```python
from build123d import *

# Parameters (mm, degrees)
BOSS_EXTRUDE1_DEPTH     = 40
CUT_EXTRUDE1_DEPTH      = 20
CUT_EXTRUDE1_DEPTH_BACK = 20
SKETCH2_R               = 1.7
BOSS_EXTRUDE2_START     = -3
SKETCH4_W               = 64
SKETCH4_H               = 30
SKETCH4_R               = 2
BOSS_EXTRUDE2_DEPTH     = 3
FILLET1_R               = 1
BOSS_EXTRUDE3_START     = -3
BOSS_EXTRUDE3_DEPTH     = 3
FILLET2_R               = 2
BOSS_EXTRUDE4_START     = -2
BOSS_EXTRUDE4_DEPTH     = 2
CHAMFER1_SIZE           = 4
CHAMFER3_SIZE           = 4
FILLET3_R               = 2


with BuildPart() as part:
    # Sketch1 → Boss-Extrude1 (new body)
    with BuildSketch(Plane.XY):
        Polygon((-3, -3), (-3, 15), (0, 15), (0, 0), (15.4, 0), (15.4, 15), (18.4, 15), (18.4, -3), align=None)
    extrude(amount=BOSS_EXTRUDE1_DEPTH)

    # Sketch2 → Cut-Extrude1 (cut, two sides: drawn at the far end of the back side and taken through both)
    with BuildSketch(Plane(origin=(0, 0, 0), x_dir=(0, 0, -1), z_dir=(1, 0, 0)).offset(-CUT_EXTRUDE1_DEPTH_BACK)):
        with Locations(Location((-34, 7.5, 0), (0, 0, 180))):
            Circle(SKETCH2_R)
        with Locations(Location((-9, 7.5, 0), (0, 0, 180))):
            Circle(SKETCH2_R)
    extrude(amount=CUT_EXTRUDE1_DEPTH + CUT_EXTRUDE1_DEPTH_BACK, mode=Mode.SUBTRACT)

    # Sketch4 → Boss-Extrude2 (add)
    with BuildSketch(Plane(origin=(0, 0, 0), x_dir=(-1, 0, 0), z_dir=(0, 0, -1)).offset(BOSS_EXTRUDE2_START)):
        with Locations((-29, -18)):
            Rectangle(SKETCH4_W, SKETCH4_H)
        with Locations((-4.875030798, -23.000128049)):
            Circle(SKETCH4_R, mode=Mode.SUBTRACT)
        with Locations((-4.87501026, -12.999951056)):
            Circle(SKETCH4_R, mode=Mode.SUBTRACT)
        with Locations((-53.124974567, -23.00004902)):
            Circle(SKETCH4_R, mode=Mode.SUBTRACT)
        with Locations((-53.125010259, -12.999787804)):
            Circle(SKETCH4_R, mode=Mode.SUBTRACT)
        with BuildLine():
            Line((-1.999964331, -28.999999992), (-55.999999981, -28.997992053))
            Line((-55.999999981, -28.997992053), (-51.282852208, -26.550624356))
            ThreePointArc((-51.282852208, -26.550624356), (-49.706744703, -25.077476419), (-49.124974567, -23.00004902))
            Line((-49.124974567, -23.00004902), (-49.125010259, -12.999787804))
            ThreePointArc((-49.125010259, -12.999787804), (-49.706039872, -10.923579364), (-51.280331003, -9.450540216))
            Line((-51.280331003, -9.450540216), (-55.999146244, -6.99799207))
            Line((-55.999146244, -6.99799207), (-1.999146282, -7.000000007))
            Line((-1.999146282, -7.000000007), (-6.718065019, -9.449859627))
            ThreePointArc((-6.718065019, -9.449859627), (-8.293505472, -10.922960328), (-8.87501026, -12.999951056))
            Line((-8.87501026, -12.999951056), (-8.875030798, -23.000128049))
            ThreePointArc((-8.875030798, -23.000128049), (-8.293584076, -25.077023205), (-6.718284054, -26.550116421))
            Line((-6.718284054, -26.550116421), (-1.999964331, -28.999999992))
        make_face(mode=Mode.SUBTRACT)
    extrude(amount=BOSS_EXTRUDE2_DEPTH)

    # Fillet1
    fillet1_edges = [part.edges().sort_by_distance(p)[0] for p in [
        (55.999999981, -28.997992053, 1.5),
        (1.999964331, -28.999999992, 1.5),
        (1.999146282, -7.000000007, 1.5),
        (55.999146244, -6.99799207, 1.5),
    ]]
    fillet(fillet1_edges, radius=FILLET1_R)

    # Sketch6 → Boss-Extrude3 (add)
    with BuildSketch(Plane(origin=(0, 0, 0), x_dir=(-1, 0, 0), z_dir=(0, 0, -1)).offset(BOSS_EXTRUDE3_START)):
        Polygon((-18.4, 15), (-61, -3), (-18.4, -3), align=None)
    extrude(amount=BOSS_EXTRUDE3_DEPTH)

    # Fillet2
    fillet2_edges = [part.edges().sort_by_distance(p)[0] for p in [
        (61, -3, 1.5),
        (-3, -33, 1.5),
        (61, -33, 1.5),
    ]]
    fillet(fillet2_edges, radius=FILLET2_R)

    # Sketch7 → Boss-Extrude4 (add)
    with BuildSketch(Plane.ZY.offset(3).offset(BOSS_EXTRUDE4_START)):
        Polygon((3, -17), (14.5, -3), (3, -3), align=None)
    extrude(amount=BOSS_EXTRUDE4_DEPTH)

    # Chamfer1
    # the kernel refuses this chamfer: 4 mm, written as the material it takes off along each edge
    with BuildSketch(Plane(origin=(28.686731952, -3, 40), x_dir=(0, -0.027495876610586403, -0.9996219169112968), z_dir=(-1, 0, 0))) as chamfer1_piece_1:
        Polygon((CHAMFER1_SIZE * 0.999621916911, -CHAMFER1_SIZE * 0.0274958766106), (-CHAMFER1_SIZE * 0.0274958766106, -CHAMFER1_SIZE * 0.999621916911), (0, 0), align=None)
    extrude(amount=41.973463904, mode=Mode.SUBTRACT)

    # Chamfer3
    chamfer3_edges = [part.edges().sort_by_distance(p)[0] for p in [
        (-1.5, 15, 0),
        (16.9, 15, 40),
        (-1.5, 15, 40),
    ]]
    chamfer(chamfer3_edges, length=CHAMFER3_SIZE)

    # Fillet3
    fillet3_edges = [part.edges().sort_by_distance(p)[0] for p in [
        (18.4, -3, 19.5),
    ]]
    fillet(fillet3_edges, radius=FILLET3_R)


solid = part.part
```
Input: part model. Units: mm. Frame: model coordinates. A direction names the side the tool comes from. Give positions to 0.01 mm unless a question says otherwise; leave off trailing zeros. Order: outer loops, then holes, each group sorted by start corner. A loop starts at its lowest first (then second) coordinate and runs counter-clockwise, first axis right, second up. Notation, with made-up numbers: (-10.75, 38.5) - (-0.75, 38.5) arc R12 cw to (-0.75, 45.5) - close; hole circle Ø11 at (25.25, 85.5). An arc over 180 degrees is marked (long way). Use a Markdown table: item, result.
(1) Section query A-A (z = 34). Output: boundary loops of the cut face in (x, y).
Computed values:
| item | result |
|---|---|
| outline | (-3, -3) - (16.4, -3) arc R2 ccw to (18.4, -1) - (18.4, 5.8) - (15.4, 5.8) - (15.4, 0) - (0, 0) - (0, 5.8) - (-3, 5.8) - close; (-3, 9.2) - (0, 9.2) - (0, 15) - (-3, 15) - close; (15.4, 9.2) - (18.4, 9.2) - (18.4, 15) - (15.4, 15) - close |
(2) Draft query along Y for faces 6 (the flat face through (15.4, 7, 20)), 7 (the flat face through (8, -1, 38)), 8 (the cylindrical face through (51.28, -13.77, 1.52)). Return one class per face: released by +Y, released by -Y, zero draft, split by the parting line, or undercut.
Computed values:
| item | result |
|---|---|
| face 6 | zero draft |
| face 7 | released by -Y |
| face 8 | undercut |
(3) Section query D-D (y = 7.5). Output: boundary loops of the cut face in (x, z).
Computed values:
| item | result |
|---|---|
| outline | (-3, 0) - (0, 0) - (0, 7.3) - (-3, 7.3) - close; (-3, 10.7) - (0, 10.7) - (0, 32.3) - (-3, 32.3) - close; (-3, 35.7) - (0, 35.7) - (0, 40) - (-3, 40) - close; (15.4, 0) - (36.15, 0) - (36.15, 3) - (18.4, 3) - (18.4, 7.3) - (15.4, 7.3) - close; (15.4, 10.7) - (18.4, 10.7) - (18.4, 32.3) - (15.4, 32.3) - close; (15.4, 35.7) - (18.4, 35.7) - (18.4, 40) - (15.4, 40) - close |
(4) Pin query (flat end, axial travel): pin 1 (17.5 mm diameter, centred on y = 10, z = 29, fed in from +X); pin 2 (4.5 mm diameter, centred on x = 4.88, y = -23, fed in from +Z); pin 3 (2 mm diameter, centred on x = 14.5, z = 14.5, fed in from -Y). Return the tip coordinate at first contact, or that it passes through.
Computed values:
| item | result |
|---|---|
| pin 1 | stops at x = 18.4 |
| pin 2 | stops at z = 3 |
| pin 3 | stops at y = -3 |
(5) Access query for faces 1 (the flat face through (-1.99, -10.1, 8.67)), 2 (the cylindrical face through (60.66, -3.21, 1.48)), 3 (the cylindrical face through (8.31, -25.05, 1.52)), 4 (the cylindrical face through (17.8, -2.43, 20.75)), 5 (the flat face through (-2, 13, 2)). Directions: +Z, -Z, +X, -X, +Y, -Y. A direction counts if a zero-diameter tool reaches every point of the face in a straight line with its end or side. Return the directions, or none.
Computed values:
| item | result |
|---|---|
| face 1 | +Z, +X, -X, -Y |
| face 2 | +Z, -Z, +X, +Y |
| face 3 | +Z, -Z |
| face 4 | +Z, +X, -Y |
| face 5 | -Z, -X, +Y |
(6) Section query B-B (y = -28). Output: boundary loops of the cut face in (x, z), then the cut area to 3 significant figures.
Computed values:
| item | result |
|---|---|
| outline | (-3, 0) - (5.1, 0) - (5.1, 3) - (-3, 3) - close; (52.9, 0) - (61, 0) - (61, 3) - (52.9, 3) - close |
| area | 48.6 mm2 |
(7) Section query C-C (x = 39.5). Output: boundary loops of the cut face in (y, z).
Computed values:
| item | result |
|---|---|
| outline | (-33, 0) - (-29, 0) - (-29, 3) - (-33, 3) - close; (-7, 0) - (6.08, 0) - (6.08, 3) - (-7, 3) - close |
(8) Line query: line 1 (X direction, y = 2.5, z = 25); line 2 (Y direction, x = -0.75, z = 9); line 3 (Z direction, x = 50, y = -12.5). Output: solid intervals per line, ascending. Write a range as from..to.
Computed values:
| item | result |
|---|---|
| line 1 | x = -3..0, 15.4..18.4 |
| line 2 | y = -3..5.8, 9.2..15 |
| line 3 | z = 0..3 |
